from build123d import *

# Parameters (mm, degrees)
BOSS_EXTRUDE1_DEPTH = 1.6
BOSS_EXTRUDE2_DEPTH = 4.4
SKETCH2_R           = 2.25
CUT_EXTRUDE1_DEPTH  = 2.75


with BuildPart() as part:
    # Sketch1 → Boss-Extrude1 (new body)
    with BuildSketch(Plane.XY):
        with BuildLine():
            Line((-4.25, 0), (-3.75, 0))
            ThreePointArc((-3.75, 0), (-2.81305998, 2.479756752), (-0.470430108, 3.720375722))
            Line((-0.470430108, 3.720375722), (-14.200896057, 1.984200385))
            ThreePointArc((-14.200896057, 1.984200385), (-15.450298656, 1.322536934), (-15.95, 0))
            Line((-15.95, 0), (-15.25, 0))
            ThreePointArc((-15.25, 0), (-14.75, 0.5), (-14.25, 0))
            Line((-14.25, 0), (-13.25, 0))
            ThreePointArc((-13.25, 0), (-12.75, 0.5), (-12.25, 0))
            Line((-12.25, 0), (-11.25, 0))
            ThreePointArc((-11.25, 0), (-10.75, 0.5), (-10.25, 0))
            Line((-10.25, 0), (-9.25, 0))
            ThreePointArc((-9.25, 0), (-8.75, 0.5), (-8.25, 0))
            Line((-8.25, 0), (-7.25, 0))
            ThreePointArc((-7.25, 0), (-6.75, 0.5), (-6.25, 0))
            Line((-6.25, 0), (-5.25, 0))
            ThreePointArc((-5.25, 0), (-4.75, 0.5), (-4.25, 0))
        make_face()
        with BuildLine():
            ThreePointArc((-0.470430108, -3.720375722), (-2.81305998, -2.479756752), (-3.75, 0))
            Line((-3.75, 0), (-4.25, 0))
            ThreePointArc((-4.25, 0), (-4.75, -0.5), (-5.25, 0))
            Line((-5.25, 0), (-6.25, 0))
            ThreePointArc((-6.25, 0), (-6.75, -0.5), (-7.25, 0))
            Line((-7.25, 0), (-8.25, 0))
            ThreePointArc((-8.25, 0), (-8.75, -0.5), (-9.25, 0))
            Line((-9.25, 0), (-10.25, 0))
            ThreePointArc((-10.25, 0), (-10.75, -0.5), (-11.25, 0))
            Line((-11.25, 0), (-12.25, 0))
            ThreePointArc((-12.25, 0), (-12.75, -0.5), (-13.25, 0))
            Line((-13.25, 0), (-14.25, 0))
            ThreePointArc((-14.25, 0), (-14.75, -0.5), (-15.25, 0))
            Line((-15.25, 0), (-15.95, 0))
            ThreePointArc((-15.95, 0), (-15.450298656, -1.322536934), (-14.200896057, -1.984200385))
            Line((-14.200896057, -1.984200385), (-0.470430108, -3.720375722))
        make_face()
        with BuildLine():
            ThreePointArc((0.470430108, 3.720375722), (2.81305998, 2.479756752), (3.75, 0))
            Line((3.75, 0), (4.25, 0))
            ThreePointArc((4.25, 0), (4.75, 0.5), (5.25, 0))
            Line((5.25, 0), (6.25, 0))
            ThreePointArc((6.25, 0), (6.75, 0.5), (7.25, 0))
            Line((7.25, 0), (8.25, 0))
            ThreePointArc((8.25, 0), (8.75, 0.5), (9.25, 0))
            Line((9.25, 0), (10.25, 0))
            ThreePointArc((10.25, 0), (10.75, 0.5), (11.25, 0))
            Line((11.25, 0), (12.25, 0))
            ThreePointArc((12.25, 0), (12.75, 0.5), (13.25, 0))
            Line((13.25, 0), (14.25, 0))
            ThreePointArc((14.25, 0), (14.75, 0.5), (15.25, 0))
            Line((15.25, 0), (15.95, 0))
            ThreePointArc((15.95, 0), (15.450298656, 1.322536934), (14.200896057, 1.984200385))
            Line((14.200896057, 1.984200385), (0.470430108, 3.720375722))
        make_face()
        with BuildLine():
            Line((4.25, 0), (3.75, 0))
            ThreePointArc((3.75, 0), (2.81305998, -2.479756752), (0.470430108, -3.720375722))
            Line((0.470430108, -3.720375722), (14.200896057, -1.984200385))
            ThreePointArc((14.200896057, -1.984200385), (15.450298656, -1.322536934), (15.95, 0))
            Line((15.95, 0), (15.25, 0))
            ThreePointArc((15.25, 0), (14.75, -0.5), (14.25, 0))
            Line((14.25, 0), (13.25, 0))
            ThreePointArc((13.25, 0), (12.75, -0.5), (12.25, 0))
            Line((12.25, 0), (11.25, 0))
            ThreePointArc((11.25, 0), (10.75, -0.5), (10.25, 0))
            Line((10.25, 0), (9.25, 0))
            ThreePointArc((9.25, 0), (8.75, -0.5), (8.25, 0))
            Line((8.25, 0), (7.25, 0))
            ThreePointArc((7.25, 0), (6.75, -0.5), (6.25, 0))
            Line((6.25, 0), (5.25, 0))
            ThreePointArc((5.25, 0), (4.75, -0.5), (4.25, 0))
        make_face()
    extrude(amount=BOSS_EXTRUDE1_DEPTH)

    # Sketch1_4 → Boss-Extrude2 (add)
    with BuildSketch(Plane.XY):
        with BuildLine():
            ThreePointArc((-1.2, 0), (0, 1.2), (1.2, 0))
            Line((1.2, 0), (3.75, 0))
            ThreePointArc((3.75, 0), (2.81305998, 2.479756752), (0.470430108, 3.720375722))
            ThreePointArc((0.470430108, 3.720375722), (0, 3.75), (-0.470430108, 3.720375722))
            ThreePointArc((-0.470430108, 3.720375722), (-2.81305998, 2.479756752), (-3.75, 0))
            Line((-3.75, 0), (-1.2, 0))
        make_face()
        with BuildLine():
            Line((3.75, 0), (1.2, 0))
            ThreePointArc((1.2, 0), (0, -1.2), (-1.2, 0))
            Line((-1.2, 0), (-3.75, 0))
            ThreePointArc((-3.75, 0), (-2.81305998, -2.479756752), (-0.470430108, -3.720375722))
            ThreePointArc((-0.470430108, -3.720375722), (0, -3.75), (0.470430108, -3.720375722))
            ThreePointArc((0.470430108, -3.720375722), (2.81305998, -2.479756752), (3.75, 0))
        make_face()
    extrude(amount=BOSS_EXTRUDE2_DEPTH)

    # Sketch2 → Cut-Extrude1 (cut)
    with BuildSketch(Plane.XY.offset(4.4)):
        Circle(SKETCH2_R)
    extrude(amount=-CUT_EXTRUDE1_DEPTH, mode=Mode.SUBTRACT)


solid = part.part
Model file for the job. Use its own axes, mm. A direction names the side the tool comes from. Round coordinates to 2 decimals unless told otherwise and drop trailing zeros. Order: outer loops, then holes, each group sorted by start corner. A loop starts at its lowest first (then second) coordinate and runs counter-clockwise, first axis right, second up.
(1) Band-saw the part on B-B (x = -8.75). List the corners of the cut face in (y, z), then the cut area to 3 significant figures.
(2) Pin check, flat tips, straight feed: pin 1 (1 mm diameter, centred on x = 4, z = 1, fed in from -Y); pin 2 (2 mm diameter, centred on x = 0, y = 0, fed in from +Z); pin 3 (2 mm diameter, centred on x = -9, y = 1, fed in from +Z). Stop position of each tip, or through.
(3) 3-axis set-ups, long thin cutter, end or side, ignore diameter. For faces 5 (the face through (-0.29, 2.23, 3.04)), 6 (the face through (15.212, 0.192, 0.789)): which of +Z, -Z, +X, -X, +Y, -Y reach the whole face in a straight line?
(4) Band-saw the part on A-A (z = 0.3). Give the number of separate pieces and of enclosed holes in the cut face, then the cut area to 3 significant figures.
(5) Drill centre lines: line 1 (Y direction, x = 0, z = 3.25); line 2 (Z direction, x = 10, y = -2); line 3 (Y direction, x = 8.5, z = 0.75). Where is each one in solid material? Low to high.
(6) Band-saw the part on C-C (z = 3.45). List the corners of the cut face in (x, y), then the cut area to 3 significant figures.
(7) Pull direction Y, two halves, no side cores. Call faces 1 (the face through (10.25, -0.02, 0.79)), 2 (the face through (-7.24, 2.864, 0.789)), 3 (the face through (7.24, -2.864, 0.789)), 4 (the face through (7.227, -0.15, 0.789)): released by +Y, released by -Y, zero draft, split by the parting line, or undercut.
(8) Band-saw the part on D-D (x = -12.75). List the corners of the cut face in (y, z), then the cut area to 3 significant figures.
Verdict:
1. outline: (-2.67, 0) - (-0.5, 0) - (-0.5, 1.6) - (-2.67, 1.6) - close; (0.5, 0) - (2.67, 0) - (2.67, 1.6) - (0.5, 1.6) - close
1. area: 6.96 mm2
2. pin 1: stops at y = -3.34
2. pin 2: passes through
2. pin 3: stops at z = 1.6
3. face 5: +Z
3. face 6: +Z, -Z
4. separate pieces: 1
4. enclosed holes: 13
4. area: 160 mm2
5. line 1: y = -3.75 to -2.25, 2.25 to 3.75
5. line 2: z = 0 to 1.6
5. line 3: y = -2.71 to -0.43, 0.43 to 2.71
6. outline: circle Ø7.5 at (0, 0); hole circle Ø4.5 at (0, 0)
6. area: 28.3 mm2
7. face 1: undercut
7. face 2: released by +Y
7. face 3: released by -Y
7. face 4: undercut
8. outline: (-2.17, 0) - (-0.5, 0) - (-0.5, 1.6) - (-2.17, 1.6) - close; (0.5, 0) - (2.17, 0) - (2.17, 1.6) - (0.5, 1.6) - close
8. area: 5.34 mm2
